Verification items for the finished model (mm, model axes). Coordinates: 2 decimals unless noted, no trailing zeros. Order: outer loops, then holes, each group sorted by start corner. A loop starts at its lowest first (then second) coordinate and runs counter-clockwise, first axis right, second up. Notation, with made-up numbers: (-31, 63.25) - (-9, 63.25) arc R19 ccw to (-9, 100.25) - close; hole circle Ø8 at (19.5, -8). An arc over 180 degrees is marked (long way). One line per question, with ' | ' between items. Start each with the question number.
from build123d import *

# Parameters (mm, degrees)
SKETCH1_R              = 15.875
SKETCH1_R_2            = 9.525
BOSS_EXTRUDE1_DEPTH    = 14.2875
CHAMFER1_SIZE          = 2
CUT_EXTRUDE1_START     = 9.191062133
CUT_EXTRUDE1_OUTLINE_R = 2.5
CUT_EXTRUDE1_DEPTH     = 6.683937969


# Read off the part's stored shape, not the designer's step: Cut-Extrude1
with BuildPart() as part:
    # Sketch1 → Boss-Extrude1 (new body)
    with BuildSketch(Plane(origin=(0, 0, 0), x_dir=(1, 0, 0), z_dir=(0, 1, 0))):
        with Locations(Location((0, 0, 0), (0, 0, 270))):
            Circle(SKETCH1_R)
        with Locations(Location((0, 0, 0), (0, 0, 270))):
            Circle(SKETCH1_R_2, mode=Mode.SUBTRACT)
    extrude(amount=BOSS_EXTRUDE1_DEPTH)

    # Chamfer1
    chamfer1_edges = [part.edges().sort_by_distance(p)[0] for p in [
        (0, 14.2875, -15.875),
    ]]
    chamfer(chamfer1_edges, length=CHAMFER1_SIZE)

    # Cut-Extrude1 outline → Cut-Extrude1 (cut)
    with BuildSketch(Plane.YZ.offset(CUT_EXTRUDE1_START)):
        with Locations((6.14375, 0)):
            Circle(CUT_EXTRUDE1_OUTLINE_R)
    extrude(amount=CUT_EXTRUDE1_DEPTH, mode=Mode.SUBTRACT)


solid = part.part
Item 1: Mould release check, pull along Z, two halves, no side actions. Record for faces 1 (the flat face through (-7, 0, 7)), 2 (the cylindrical face through (12.49, 8.53, 0.75)), 3 (the cylindrical face through (-15.497, 6.058, -3.441)): +Z half, -Z half, draft (parallel to the pull), parting line (faces both ways), or undercut.
Item 2: Thickness scan on probe 1 along Y at (x, z) = (11, 0); probe 2 along X at (y, z) = (10.5, 0) (3 decimals); probe 3 along Z at (x, y) = (-7.5, 12.5). Record the ranges inside material, lowest first. Write a range as from..to.
Item 3: Section check A-A (z = 0). Record the cut outline in (x, y) (1 decimal), then the cut area to 3 significant figures.
Item 4: Gauge pin test, flat end, axial feed: pin 1 (3 mm diameter, centred on y = 7.5, z = -7.5, fed in from +X). Record the tip position at first contact, or that the pin passes through.
Item 5: Section check D-D (y = 7.5). Record the cut outline in (x, z) (3 decimals), then the cut area to 3 significant figures.
Item 6: Section check C-C (y = 3). Record the cut outline in (x, z) (3 decimals), then the cut area to 3 significant figures.
Item 7: Section check B-B (x = 0). Record the cut outline in (y, z) (1 decimal).
Completed:
1) face 1: draft | face 2: undercut | face 3: parting line
2) probe 1: y = 0..3.64, 8.64..14.29 | probe 2: x = -15.875..-9.525, 9.525..15.875 | probe 3: z = -13.75..-5.87, 5.87..13.75
3) outline: (-15.9, 0) - (-9.5, 0) - (-9.5, 14.3) - (-13.9, 14.3) - (-15.9, 12.3) - close; (9.5, 0) - (15.9, 0) - (15.9, 3.6) - (9.5, 3.6) - close; (9.5, 8.6) - (15.9, 8.6) - (15.9, 12.3) - (13.9, 14.3) - (9.5, 14.3) - close | area: 146 mm^2
4) pin 1: stops at x = 14.7
5) outline: (9.291, -2.1) arc R9.525 cw (long way) to (9.291, 2.1) - (15.735, 2.1) arc R15.875 ccw (long way) to (15.735, -2.1) - close | area: 480 mm^2
6) outline: circle Ø31.75 at (0, 0); hole circle Ø19.05 at (0, 0) | area: 507 mm^2
7) outline: (0, -15.9) - (12.3, -15.9) - (14.3, -13.9) - (14.3, -9.5) - (0, -9.5) - close; (0, 9.5) - (14.3, 9.5) - (14.3, 13.9) - (12.3, 15.9) - (0, 15.9) - close
